```python
from build123d import *

# Parameters (mm, degrees)
BOSS_EXTRUDE1_DEPTH        = 14
M3_CLEARANCE_HOLE1_REACH   = 33.048
M3_CLEARANCE_HOLE1_BORE_R  = 1.6
M2X0_4_TAPPED_HOLE1_REACH  = 33.048
M2X0_4_TAPPED_HOLE1_BORE_R = 0.8


with BuildPart() as part:
    # Sketch1 → Boss-Extrude1 (new body)
    with BuildSketch(Plane.XY):
        Polygon((12, 6.92820323), (0, 13.856406461), (-12, 6.92820323), (-12, -6.92820323), (0, -13.856406461), (12, -6.92820323), align=None)
        with BuildLine():
            ThreePointArc((-2.5, -7.599342077), (-8, 0), (-2.5, 7.599342077))
            Line((-2.5, 7.599342077), (-2.5, 10.3))
            Line((-2.5, 10.3), (2.5, 10.3))
            Line((2.5, 10.3), (2.5, 7.599342077))
            ThreePointArc((2.5, 7.599342077), (6.480740698, 4.69041576), (8, 0))
            ThreePointArc((8, 0), (6.480740698, -4.69041576), (2.5, -7.599342077))
            Line((2.5, -7.599342077), (2.5, -10.3))
            Line((2.5, -10.3), (-2.5, -10.3))
            Line((-2.5, -10.3), (-2.5, -7.599342077))
        make_face(mode=Mode.SUBTRACT)
    extrude(amount=BOSS_EXTRUDE1_DEPTH)

    # M3 Clearance Hole1 bore → M3 Clearance Hole1 (cut, up to next)
    with BuildSketch(Plane(origin=(12, 0, 0), x_dir=(0, 0, -1), z_dir=(1, 0, 0)), mode=Mode.PRIVATE) as m3_clearance_hole1_sk1:
        with Locations((-9.5, 0)):
            Circle(M3_CLEARANCE_HOLE1_BORE_R)
    m3_clearance_hole1_tool1 = extrude(m3_clearance_hole1_sk1.sketch, amount=-M3_CLEARANCE_HOLE1_REACH, mode=Mode.PRIVATE) & part.part
    add(m3_clearance_hole1_tool1.solids().sort_by_distance((12, 0, 9.5))[0], mode=Mode.SUBTRACT)

    # M2x0.4 Tapped Hole1 bore → M2x0.4 Tapped Hole1 (cut, up to next)
    with BuildSketch(Plane.ZY.offset(12), mode=Mode.PRIVATE) as m2x0_4_tapped_hole1_sk1:
        with Locations((2, 0)):
            Circle(M2X0_4_TAPPED_HOLE1_BORE_R)
    m2x0_4_tapped_hole1_tool1 = extrude(m2x0_4_tapped_hole1_sk1.sketch, amount=-M2X0_4_TAPPED_HOLE1_REACH, mode=Mode.PRIVATE) & part.part
    add(m2x0_4_tapped_hole1_tool1.solids().sort_by_distance((-12, 0, 2))[0], mode=Mode.SUBTRACT)


solid = part.part
```
Could you check a few things on this model? Use its own coordinates, in mm. A direction names the side the tool comes from. Give positions to 0.01 mm unless a question says otherwise; leave off trailing zeros. Write each loop counter-clockwise with the first axis right and the second up, starting at its lowest first coordinate (ties: lowest second). Pieces come first, ordered by that corner, then holes. Notation, with made-up numbers: (69.5, 49.5) - (110.5, 49.5) arc R13 ccw to (110.5, 57.5) - close; hole circle Ø2 at (-18.75, 85). An arc over 180 degrees is marked (long way). One line per item, written item: value. Start each with the question number.
Item 1: Imagine slicing it at D-D, the plane z = 4. List the corners of the cut face in (x, y) for me.
Item 2: Imagine slicing it at C-C, the plane y = -9.5. List the corners of the cut face in (x, z) for me.
Item 3: I'm going to push flat-ended pins straight in: pin 1 (2.5 mm diameter, centred on x = -0.5, z = 6, fed in from -Y); pin 2 (5 mm diameter, centred on x = -9.5, z = 7.5, fed in from -Y); pin 3 (0.8 mm diameter, centred on y = -8.5, z = 6, fed in from -X); pin 4 (8 mm diameter, centred on x = 4.5, y = 1.5, fed in from +Z). Where does each tip first touch, or does it pass through?
Item 4: Which directions (+Z, -Z, +X, -X, +Y, -Y) give clear straight access to the entire face, cutting with the end or side of a thin tool? Please do faces 5 (the face through (-10.008, -0.306, 2.739)), 6 (the face through (2.5, 9, 7)), 7 (the face through (-6, -6, 0)), 8 (the face through (9.95, 0.07, 11.1)).
Item 5: If we mould it in two halves opening along X, with no side actions, what happens to faces 1 (the face through (2.5, -9, 7)), 2 (the face through (-8, 0, 7)), 3 (the face through (-6, -6, 14)), 4 (the face through (6.084, 10.344, 6.902))? For each: +X half, -X half, draft (parallel to the pull), parting line (faces both ways), or undercut.
Item 6: Imagine slicing it at A-A, the plane z = 2. List the corners of the cut face in (x, y) for me, and give its area (3 significant figures).
Item 7: Imagine slicing it at B-B, the plane x = 3.5. List the corners of the cut face in (y, z) for me.
Item 8: Please list where these lines run through material, in increasing order: line 1 (X direction, y = -4, z = 13.25); line 2 (Y direction, x = -5, z = 10) (3 decimals); line 3 (Y direction, x = -3.25, z = 5). Write a range as from..to.
Geometry says:
1. outline: (-12, -6.93) - (0, -13.86) - (12, -6.93) - (12, 6.93) - (0, 13.86) - (-12, 6.93) - close; hole (-2.5, -10.3) - (2.5, -10.3) - (2.5, -7.6) arc R8 ccw to (2.5, 7.6) - (2.5, 10.3) - (-2.5, 10.3) - (-2.5, 7.6) arc R8 ccw to (-2.5, -7.6) - close
2. outline: (-7.55, 0) - (-2.5, 0) - (-2.5, 14) - (-7.55, 14) - close; (2.5, 0) - (7.55, 0) - (7.55, 14) - (2.5, 14) - close
3. pin 1: y = -13.86
3. pin 2: y = -9.81
3. pin 3: x = -9.97
3. pin 4: z = 14
4. face 5: -X
4. face 6: +Z, -Z
4. face 7: -Z, +X, -X, +Y, -Y
4. face 8: +X
5. face 1: undercut
5. face 2: undercut
5. face 3: draft
5. face 4: +X half
6. outline: (-12, -6.93) - (0, -13.86) - (12, -6.93) - (12, 6.93) - (0, 13.86) - (-12, 6.93) - (-12, 0.8) - (-7.96, 0.8) arc R8 cw to (-2.5, 7.6) - (-2.5, 10.3) - (2.5, 10.3) - (2.5, 7.6) arc R8 cw to (2.5, -7.6) - (2.5, -10.3) - (-2.5, -10.3) - (-2.5, -7.6) arc R8 cw to (-7.96, -0.8) - (-12, -0.8) - close
6. area: 267 mm^2
7. outline: (-11.84, 0) - (-7.19, 0) - (-7.19, 14) - (-11.84, 14) - close; (7.19, 0) - (11.84, 0) - (11.84, 14) - (7.19, 14) - close
8. line 1: -12..-6.93, 6.93..12
8. line 2: -10.97..-6.245, 6.245..10.97
8. line 3: -11.98..-7.31, 7.31..11.98
